Geometry: final body of the model. Coordinates: model frame, mm. Face numbers are marked on the shaded views. Coordinates: 2 decimals unless noted, no trailing zeros. Loops run counter-clockwise (first coordinate to the right, second up) from the corner with the lowest first, then second, coordinate; pieces in that order, holes last. Notation, with made-up numbers: (-37, 42) -> (15, 42) arc R19 cw to (15, 72) -> close; hole circle Ø5 at (35, 86). An arc over 180 degrees is marked (long way). One line per item, written item: value. Start each with the question number.
Item 1: Mould query, pull axis Y, two halves, no side actions, for the marked faces 1, 2 and 3. Classes: +Y half, -Y half, draft (parallel to the pull), parting line (faces both ways), or undercut.
Item 2: Section query A-A on x = 0. Return loops of the section in (y, z) (3 decimals).
Item 3: Ray query, probe 1 along Z at (x, y) = (0, -13.75) (3 decimals); probe 2 along Y at (x, z) = (0, 1.55); probe 3 along Y at (x, z) = (-0.25, -1.5) (3 decimals). Return the intervals inside material, ascending. Write a range as from..to.
Item 4: Section query B-B on z = 0. Return loops of the section in (x, y) (3 decimals).
Item 5: Section query D-D on x = -2.5. Return loops of the section in (y, z) (3 decimals).
Item 6: Contact query for flat-ended pins moving along their axis: pin 1 Ø1.5 at (y, z) = (-7.5, -1) entering from -X; pin 2 Ø1.5 at (x, y) = (2.5, -12) entering from -Z; pin 3 Ø1.5 at (y, z) = (6.5, -2.5) entering from +X; pin 4 Ø1.2 at (x, z) = (0, 0) entering from -Y (3 decimals). Output: stop coordinate, or through.
Item 7: Section query C-C on y = 11.5. Return loops of the section in (x, z) (3 decimals), then the cut area to 3 significant figures.
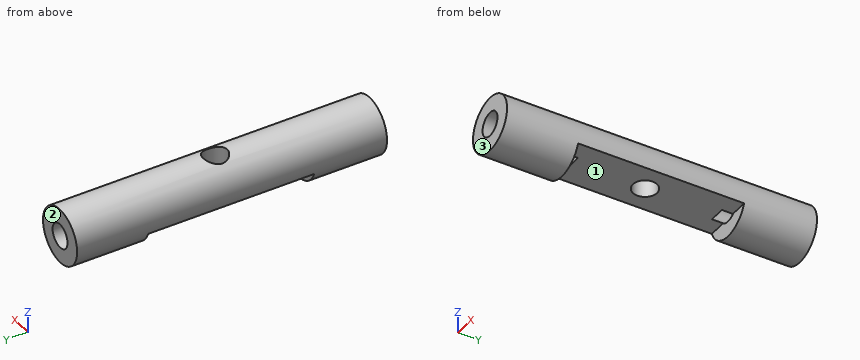
from build123d import *

# Parameters (mm, degrees)
F0_R     = 3.175
F1_DEPTH = 17.78
F2_R     = 1.3890625
F3_DEPTH = 9.525
F4_R     = 1.3890625
F5_DEPTH = 9.525
F6_W     = 19.05
F6_H     = 2.159
F7_DEPTH = 9.525
F8_R     = 1.3890625
F9_DEPTH = 3.175


with BuildPart() as f1:
    # F0 (on Front) → F1 (new body, symmetric)
    with BuildSketch(Plane.XZ):
        Circle(F0_R)
    extrude(amount=F1_DEPTH, both=True)

    # F2 (on face) → F3 (cut)
    with BuildSketch(Plane.XZ.offset(17.78)):
        Circle(F2_R)
    extrude(amount=-F3_DEPTH, mode=Mode.SUBTRACT)

    # F4 (on face) → F5 (cut)
    with BuildSketch(Plane(origin=(0, 17.78, 0), x_dir=(-1, 0, 0), z_dir=(0, 1, 0))):
        Circle(F4_R)
    extrude(amount=-F5_DEPTH, mode=Mode.SUBTRACT)

    # F6 (on Front) → F7 (cut, symmetric)
    with BuildSketch(Plane.XZ):
        with Locations((-0.3555464804, -2.1219391367)):
            Rectangle(F6_W, F6_H)
    extrude(amount=F7_DEPTH, both=True, mode=Mode.SUBTRACT)

    # F8 (on Top) → F9 (cut, symmetric)
    with BuildSketch(Plane.XY):
        Circle(F8_R)
    extrude(amount=F9_DEPTH, both=True, mode=Mode.SUBTRACT)


solid = f1.part
Reply:
1. face 1: undercut
1. face 2: +Y half
1. face 3: -Y half
2. outline: (-17.78, -3.175) -> (-9.525, -3.175) -> (-9.525, -1.389) -> (-17.78, -1.389) -> close; (-17.78, 1.389) -> (-8.255, 1.389) -> (-8.255, -1.042) -> (-1.389, -1.042) -> (-1.389, 3.175) -> (-17.78, 3.175) -> close; (1.389, -1.042) -> (8.255, -1.042) -> (8.255, 1.389) -> (17.78, 1.389) -> (17.78, 3.175) -> (1.389, 3.175) -> close; (9.525, -3.175) -> (17.78, -3.175) -> (17.78, -1.389) -> (9.525, -1.389) -> close
3. probe 1: z = -3.175..-1.389, 1.389..3.175
3. probe 2: y = -17.78..-1.39, 1.39..17.78
3. probe 3: y = -17.78..-9.525, 9.525..17.78
4. outline: (-3.175, -17.78) -> (-1.389, -17.78) -> (-1.389, -8.255) -> (1.389, -8.255) -> (1.389, -17.78) -> (3.175, -17.78) -> (3.175, 17.78) -> (1.389, 17.78) -> (1.389, 8.255) -> (-1.389, 8.255) -> (-1.389, 17.78) -> (-3.175, 17.78) -> close; hole circle Ø2.778 at (0, 0)
5. outline: (-17.78, -1.957) -> (-9.525, -1.957) -> (-9.525, -1.042) -> (9.525, -1.042) -> (9.525, -1.957) -> (17.78, -1.957) -> (17.78, 1.957) -> (-17.78, 1.957) -> close
6. pin 1: stops at x = -3.17
6. pin 2: stops at z = -2.65
6. pin 3: passes through
6. pin 4: stops at y = -8.255
7. outline: circle Ø6.35 at (0, 0); hole circle Ø2.778 at (0, 0)
7. area: 25.6 mm²
